from build123d import *

# Parameters (mm, degrees)
PAD_DEPTH = 10


with BuildPart() as part:
    # Sketch → Pad (new body)
    with BuildSketch(Plane.XY):
        with BuildLine():
            Line((30, 0), (30, 30))
            Line((30, 30), (0, 30))
            Line((0, 30), (0, 31))
            Line((0, 31), (30, 31))
            ThreePointArc((32, 30), (31.809017, 32.118034), (30, 31))
            Line((32, 30), (32, 0))
            Line((32, 0), (30, 0))
        make_face()
    extrude(amount=PAD_DEPTH)


solid = part.part
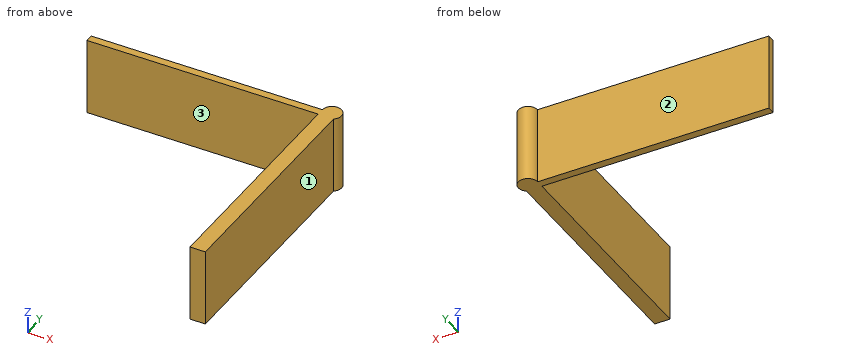
Geometry: final body of the model. Coordinates: model frame, mm. Face numbers are marked on the shaded views. A direction names the side the tool comes from. Coordinates: 2 decimals unless noted, no trailing zeros. Loops run counter-clockwise (first coordinate to the right, second up) from the corner with the lowest first, then second, coordinate; pieces in that order, holes last. Notation, with made-up numbers: (12, 49) - (42, 49) arc R25 ccw to (42, 75) - close; hole circle Ø5 at (-37, 17). An arc over 180 degrees is marked (long way). One line per question, with ' | ' between items. Start each with the question number.
(1) Reachability of the marked faces 1, 2 and 3 from +Z, -Z, +X, -X, +Y, -Y: full face, straight path, thin tool, end or side. Return the list, or none.
(2) Cut plane A-A on z = 9.25. Output: boundary loops of the cut face in (x, y).
(3) Ray query, L1, parallel to Y at x = 8.5, z = 6.75; L2, parallel to X at y = 21.5, z = 9.5. Return the intervals inside material, ascending. Write a range as from..to.
(4) Cut plane B-B on x = 24.5. Output: boundary loops of the cut face in (y, z).
(5) Cut plane C-C on y = 17.5. Output: boundary loops of the cut face in (x, z), and give its area (3 significant figures).
(6) First-contact query: pin 1 (5 mm diameter, centred on x = 3.5, z = 6.5, fed in from +Y); pin 2 (5 mm diameter, centred on y = 10.5, z = 3.5, fed in from -X); pin 3 (1 mm diameter, centred on y = 21, z = 4, fed in from +X). Flat tips, straight axial feed; report the tip coordinate or a pass-through.
Here are the results:
1) face 1: +Z, -Z, +X, -Y | face 2: +Z, -Z, -X, +Y | face 3: +Z, -Z, -X, -Y
2) outline: (0, 30) - (30, 30) - (30, 0) - (32, 0) - (32, 30) arc R1.25 ccw (long way) to (30, 31) - (0, 31) - close
3) L1: 30..31 | L2: 30..32
4) outline: (30, 0) - (31, 0) - (31, 10) - (30, 10) - close
5) outline: (30, 0) - (32, 0) - (32, 10) - (30, 10) - close | area: 20.0 mm²
6) pin 1: y = 31 | pin 2: x = 30 | pin 3: x = 32
